Drawing for the job (mm, zero at the part's lowest x, y, z). A direction names the side the tool comes from. Give positions to 0.01 mm unless a question says otherwise; leave off trailing zeros. Loops run counter-clockwise (first coordinate to the right, second up) from the corner with the lowest first, then second, coordinate; pieces in that order, holes last. Notation, with made-up numbers: (35.5, 5) -> (70.5, 5) arc R18 ccw to (70.5, 24) -> close; hole circle Ø4 at (14.5, 40). An arc over 180 degrees is marked (long way). Answer in a Markdown table with one row per item. Add a question column.
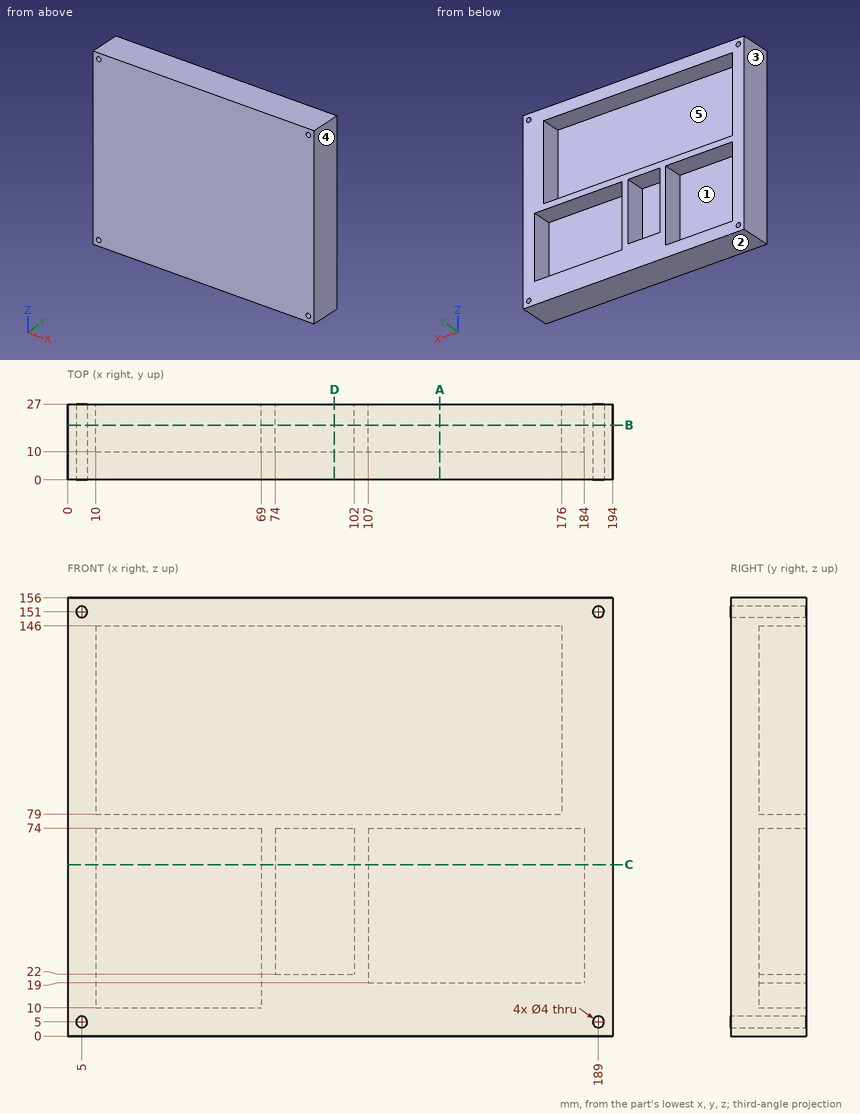
(1) 3-axis set-ups, long thin cutter, end or side, ignore diameter. For the marked faces 4 and 5: which of +Z, -Z, +X, -X, +Y, -Y reach the whole face in a straight line?
(2) Flat gauge pins, fed straight in: pin 1 Ø3.5 at (x, z) = (189, 151) entering from +Y; pin 2 Ø3 at (y, z) = (23, 23.5) entering from -X; pin 3 Ø5 at (x, z) = (123.5, 100) entering from +Y. Where does each tip first touch, or does it go through?
(3) Wall check: line 1 along Z through (x, y) = (87, 25); line 2 along X through (y, z) = (15.5, 151); line 3 along Z through (x, y) = (126, 11.75). Give the ranges that are in metal, low to high. Write a range as from..to.
(4) Saw through at D-D, the plane x = 95. List the corners of the cut face in (y, z).
(5) Saw through at C-C, the plane z = 61. List the corners of the cut face in (x, y).
(6) Saw through at A-A, the plane x = 132.5. List the corners of the cut face in (y, z), then the cut area to 3 significant figures.
(7) Two-plate mould, pull along Z, no slides. Class the marked faces 1, 2 and 3: released by +Z, released by -Z, zero draft, split by the parting line, or undercut.
(8) Saw through at B-B, the plane y = 19.5. State how many separate pieces and enclosed holes the cut face has, then the cut area to 3 significant figures.
Worked answers:
| question | item | result |
|---|---|---|
| 1 | face 4 | +Z, -Z, +X, +Y, -Y |
| 1 | face 5 | +Y |
| 2 | pin 1 | through |
| 2 | pin 2 | x = 0 |
| 2 | pin 3 | y = 10 |
| 3 | line 1 | 0..22, 74..79, 146..156 |
| 3 | line 2 | 0..3, 7..187, 191..194 |
| 3 | line 3 | 0..19, 74..79, 146..156 |
| 4 | outline | (0, 0) -> (27, 0) -> (27, 22) -> (10, 22) -> (10, 74) -> (27, 74) -> (27, 79) -> (10, 79) -> (10, 146) -> (27, 146) -> (27, 156) -> (0, 156) -> close |
| 5 | outline | (0, 0) -> (194, 0) -> (194, 27) -> (184, 27) -> (184, 10) -> (107, 10) -> (107, 27) -> (102, 27) -> (102, 10) -> (74, 10) -> (74, 27) -> (69, 27) -> (69, 10) -> (10, 10) -> (10, 27) -> (0, 27) -> close |
| 6 | outline | (0, 0) -> (27, 0) -> (27, 19) -> (10, 19) -> (10, 74) -> (27, 74) -> (27, 79) -> (10, 79) -> (10, 146) -> (27, 146) -> (27, 156) -> (0, 156) -> close |
| 6 | area | 2,140 mm^2 |
| 7 | face 1 | undercut |
| 7 | face 2 | released by -Z |
| 7 | face 3 | zero draft |
| 8 | separate pieces | 1 |
| 8 | enclosed holes | 8 |
| 8 | area | 9,620 mm^2 |
